Can you work these out from the model? Positions are in its coordinate system, mm. Coordinates: 2 decimals unless noted, no trailing zeros. Return JSON: item names as keys, results as strings. Group by question number.
1) For pin 1 Ø10 at (x, y) = (33.5, 26) entering from -Z; pin 2 Ø8 at (y, z) = (6, 452.5) entering from +X; pin 3 Ø13 at (x, z) = (-11, 514) entering from -Y, each with a flat end and sliding along its axis, tell me the tip position at first contact or that it passes through.
2) If I drill on line 1 along X through (y, z) = (-39, 925); line 2 along Y through (x, z) = (-5, 936.5); line 3 along Y through (x, z) = (28, 216.5), over which ranges is the centre line in solid material (lowest first)?
3) Imagine slicing it at A-A (z = 875). Give the number of separate pieces and of enclosed holes in the cut face, and give its area (3 significant figures).
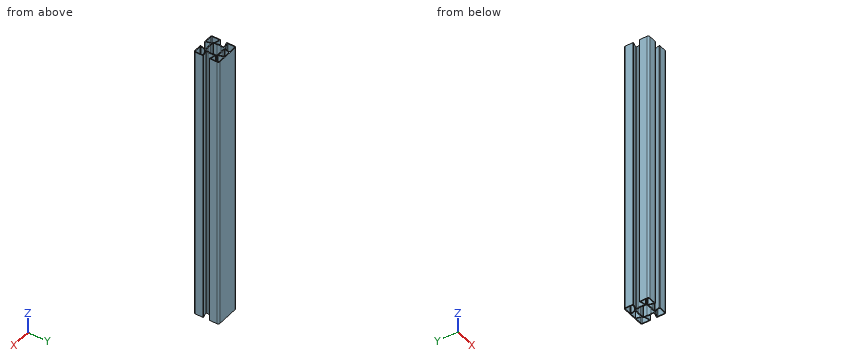
```python
from build123d import *

# Parameters (mm, degrees)
F1_DEPTH = 1000


# Not quite as in the source:
# - ends of sketch curves that miss each other by under 0.0002 mm in the source are joined


with BuildPart() as f1:
    # F0 (on Top) → F1 (new body)
    with BuildSketch(Plane.XY):
        with BuildLine():
            ThreePointArc((8.8614578186, -23.0888885991), (9.062799833, -23.022474706), (9.273618, -23))
            Line((9.273618, -23), (14.841657, -23))
            ThreePointArc((14.841657, -23), (15.6350103133, -23.3912385359), (15.8075828492, -24.2588189596))
            Line((15.8075828492, -24.2588189596), (10.671624, -43.426476))
            ThreePointArc((10.671624, -43.426476), (10.8873403242, -44.5109517857), (11.879032, -45))
            Line((11.879032, -45), (39, -45))
            ThreePointArc((39, -45), (43.2426406871, -43.2426406871), (45, -39))
            Line((45, -39), (45, -11.879032))
            ThreePointArc((45, -11.879032), (44.5109517857, -10.8873403242), (43.4264761923, -10.6716247175))
            Line((43.4264761923, -10.6716247175), (24.258819, -15.807583))
            ThreePointArc((24.258819, -15.807583), (23.3912385359, -15.6350103133), (23, -14.841657))
            Line((23, -14.841657), (23, -9.273618))
            ThreePointArc((23, -9.273618), (23.022474706, -9.062799833), (23.0888885991, -8.8614578186))
            ThreePointArc((23.0888885991, -8.8614578186), (25, 0), (23.0888887851, 8.8614579028))
            ThreePointArc((23.0888887851, 8.8614579028), (23.022474706, 9.062799833), (23, 9.273618))
            Line((23, 9.273618), (23, 14.841657))
            ThreePointArc((23, 14.841657), (23.3912385359, 15.6350103133), (24.2588189596, 15.8075828492))
            Line((24.2588189596, 15.8075828492), (43.426476, 10.671624))
            ThreePointArc((43.426476, 10.671624), (44.5109517857, 10.8873403242), (45, 11.879032))
            Line((45, 11.879032), (45, 39))
            ThreePointArc((45, 39), (43.2426406871, 43.2426406871), (39, 45))
            Line((39, 45), (-39, 45))
            ThreePointArc((-39, 45), (-43.2426406871, 43.2426406871), (-45, 39))
            Line((-45, 39), (-45, 11.879032))
            ThreePointArc((-45, 11.879032), (-44.5109517857, 10.8873403242), (-43.4264761923, 10.6716247175))
            Line((-43.4264761923, 10.6716247175), (-24.258819, 15.807583))
            ThreePointArc((-24.258819, 15.807583), (-23.3912385359, 15.6350103133), (-23, 14.841657))
            Line((-23, 14.841657), (-23, 9.273618))
            ThreePointArc((-23, 9.273618), (-23.022474706, 9.062799833), (-23.0888885991, 8.8614578186))
            ThreePointArc((-23.0888885991, 8.8614578186), (-25, 0), (-23.0888887851, -8.8614579028))
            ThreePointArc((-23.0888887851, -8.8614579028), (-23.022474706, -9.062799833), (-23, -9.273618))
            Line((-23, -9.273618), (-23, -14.841657))
            ThreePointArc((-23, -14.841657), (-23.3912385359, -15.6350103133), (-24.2588189596, -15.8075828492))
            Line((-24.2588189596, -15.8075828492), (-43.426476, -10.671624))
            ThreePointArc((-43.426476, -10.671624), (-44.5109517857, -10.8873403242), (-45, -11.879032))
            Line((-45, -11.879032), (-45, -39))
            ThreePointArc((-45, -39), (-43.2426406871, -43.2426406871), (-39, -45))
            Line((-39, -45), (-11.879032, -45))
            ThreePointArc((-11.879032, -45), (-10.8873403242, -44.5109517857), (-10.6716247175, -43.4264761923))
            Line((-10.6716247175, -43.4264761923), (-15.807583, -24.258819))
            ThreePointArc((-15.807583, -24.258819), (-15.6350103133, -23.3912385359), (-14.841657, -23))
            Line((-14.841657, -23), (-9.273618, -23))
            ThreePointArc((-9.273618, -23), (-9.062799833, -23.022474706), (-8.8614578186, -23.0888885991))
            ThreePointArc((-8.8614578186, -23.0888885991), (0, -25), (8.8614578186, -23.0888885991))
        make_face()
        with BuildLine():
            Line((-39.732362, -14.508469), (-24.482362, -18.594694))
            ThreePointArc((-24.482362, -18.594694), (-23.4132933733, -19.3090230718), (-23, -20.526546))
            Line((-23, -20.526546), (-23, -21))
            ThreePointArc((-23, -21), (-22.4142135624, -22.4142135624), (-21, -23))
            Line((-21, -23), (-20.526546, -23))
            ThreePointArc((-20.526546, -23), (-19.3090230718, -23.4132933733), (-18.5946943016, -24.4823620808))
            Line((-18.5946943016, -24.4823620808), (-14.508469, -39.732362))
            ThreePointArc((-14.508469, -39.732362), (-14.8536143733, -41.4675229282), (-16.440321, -42.25))
            Line((-16.440321, -42.25), (-39, -42.25))
            ThreePointArc((-39, -42.25), (-41.2980970389, -41.2980970389), (-42.25, -39))
            Line((-42.25, -39), (-42.25, -16.440321))
            ThreePointArc((-42.25, -16.440321), (-41.4675229282, -14.8536143733), (-39.732362, -14.508469))
        make_face(mode=Mode.SUBTRACT)
        with BuildLine():
            Line((14.508469, -39.732362), (18.594694, -24.482362))
            ThreePointArc((18.594694, -24.482362), (19.3090230718, -23.4132933733), (20.526546, -23))
            Line((20.526546, -23), (21, -23))
            ThreePointArc((21, -23), (22.4142135624, -22.4142135624), (23, -21))
            Line((23, -21), (23, -20.526546))
            ThreePointArc((23, -20.526546), (23.4132933733, -19.3090230718), (24.4823620808, -18.5946943016))
            Line((24.4823620808, -18.5946943016), (39.732362, -14.508469))
            ThreePointArc((39.732362, -14.508469), (41.4675229282, -14.8536143733), (42.25, -16.440321))
            Line((42.25, -16.440321), (42.25, -39))
            ThreePointArc((42.25, -39), (41.2980970389, -41.2980970389), (39, -42.25))
            Line((39, -42.25), (16.440321, -42.25))
            ThreePointArc((16.440321, -42.25), (14.8536143733, -41.4675229282), (14.508469, -39.732362))
        make_face(mode=Mode.SUBTRACT)
        with BuildLine():
            Line((-7.3951, -20.25), (-19.25, -20.25))
            ThreePointArc((-19.25, -20.25), (-19.9571067812, -19.9571067812), (-20.25, -19.25))
            Line((-20.25, -19.25), (-20.25, -7.3951))
            ThreePointArc((-20.25, -7.3951), (-20.2639867072, -7.2284333074), (-20.3055555728, -7.0664288513))
            ThreePointArc((-20.3055554887, -7.066428822), (-21.5, 0), (-20.3055554887, 7.066428822))
            ThreePointArc((-20.3055555728, 7.0664288513), (-20.2639867072, 7.2284333074), (-20.25, 7.3951))
            Line((-20.25, 7.3951), (-20.25, 19.25))
            ThreePointArc((-20.25, 19.25), (-19.9571067812, 19.9571067812), (-19.25, 20.25))
            Line((-19.25, 20.25), (-7.3951, 20.25))
            ThreePointArc((-7.3951, 20.25), (-7.2284333074, 20.2639867072), (-7.0664288513, 20.3055555728))
            ThreePointArc((-7.066428822, 20.3055554887), (0, 21.5), (7.066428822, 20.3055554887))
            ThreePointArc((7.0664288513, 20.3055555728), (7.2284333074, 20.2639867072), (7.3951, 20.25))
            Line((7.3951, 20.25), (19.25, 20.25))
            ThreePointArc((19.25, 20.25), (19.9571067812, 19.9571067812), (20.25, 19.25))
            Line((20.25, 19.25), (20.25, 7.3951))
            ThreePointArc((20.25, 7.3951), (20.2639867072, 7.2284333074), (20.3055555728, 7.0664288513))
            ThreePointArc((20.3055554887, 7.066428822), (21.5, 0), (20.3055554887, -7.066428822))
            ThreePointArc((20.3055555728, -7.0664288513), (20.2639867072, -7.2284333074), (20.25, -7.3951))
            Line((20.25, -7.3951), (20.25, -19.25))
            ThreePointArc((20.25, -19.25), (19.9571067812, -19.9571067812), (19.25, -20.25))
            Line((19.25, -20.25), (7.3951, -20.25))
            ThreePointArc((7.3951, -20.25), (7.2284333074, -20.2639867072), (7.0664288513, -20.3055555728))
            ThreePointArc((7.066428822, -20.3055554887), (0, -21.5), (-7.066428822, -20.3055554887))
            ThreePointArc((-7.0664288513, -20.3055555728), (-7.2284333074, -20.2639867072), (-7.3951, -20.25))
        make_face(mode=Mode.SUBTRACT)
        with BuildLine():
            Line((-14.508469, 39.732362), (-18.594694, 24.482362))
            ThreePointArc((-18.594694, 24.482362), (-19.3090230718, 23.4132933733), (-20.526546, 23))
            Line((-20.526546, 23), (-21, 23))
            ThreePointArc((-21, 23), (-22.4142135624, 22.4142135624), (-23, 21))
            Line((-23, 21), (-23, 20.526546))
            ThreePointArc((-23, 20.526546), (-23.4132933733, 19.3090230718), (-24.4823620808, 18.5946943016))
            Line((-24.4823620808, 18.5946943016), (-39.732362, 14.508469))
            ThreePointArc((-39.732362, 14.508469), (-41.4675229282, 14.8536143733), (-42.25, 16.440321))
            Line((-42.25, 16.440321), (-42.25, 39))
            ThreePointArc((-42.25, 39), (-41.2980970389, 41.2980970389), (-39, 42.25))
            Line((-39, 42.25), (-16.440321, 42.25))
            ThreePointArc((-16.440321, 42.25), (-14.8536143733, 41.4675229282), (-14.508469, 39.732362))
        make_face(mode=Mode.SUBTRACT)
        with BuildLine():
            Line((-9.273618, 23), (-14.841657, 23))
            ThreePointArc((-14.841657, 23), (-15.6350103133, 23.3912385359), (-15.8075828492, 24.2588189596))
            Line((-15.8075828492, 24.2588189596), (-10.98686, 42.25))
            Line((-10.98686, 42.25), (10.98686, 42.25))
            Line((10.98686, 42.25), (15.807583, 24.258819))
            ThreePointArc((15.807583, 24.258819), (15.6350103133, 23.3912385359), (14.841657, 23))
            Line((14.841657, 23), (9.273618, 23))
            ThreePointArc((9.273618, 23), (9.062799833, 23.022474706), (8.8614578186, 23.0888885991))
            ThreePointArc((8.8614578186, 23.0888885991), (0, 25), (-8.8614579028, 23.0888887851))
            ThreePointArc((-8.8614579028, 23.0888887851), (-9.062799833, 23.022474706), (-9.273618, 23))
        make_face(mode=Mode.SUBTRACT)
        with BuildLine():
            Line((39.732362, 14.508469), (24.482362, 18.594694))
            ThreePointArc((24.482362, 18.594694), (23.4132933733, 19.3090230718), (23, 20.526546))
            Line((23, 20.526546), (23, 21))
            ThreePointArc((23, 21), (22.4142135624, 22.4142135624), (21, 23))
            Line((21, 23), (20.526546, 23))
            ThreePointArc((20.526546, 23), (19.3090230718, 23.4132933733), (18.5946943016, 24.4823620808))
            Line((18.5946943016, 24.4823620808), (14.508469, 39.732362))
            ThreePointArc((14.508469, 39.732362), (14.8536143733, 41.4675229282), (16.440321, 42.25))
            Line((16.440321, 42.25), (39, 42.25))
            ThreePointArc((39, 42.25), (41.2980970389, 41.2980970389), (42.25, 39))
            Line((42.25, 39), (42.25, 16.440321))
            ThreePointArc((42.25, 16.440321), (41.4675229282, 14.8536143733), (39.732362, 14.508469))
        make_face(mode=Mode.SUBTRACT)
    extrude(amount=F1_DEPTH)


solid = f1.part
```
Calculated:
{
 "1": {"pin 1": "through", "pin 2": "x = 24.91", "pin 3": "y = -45"},
 "2": {"line 1": "-45 to -42.25, -14.7 to -11.86, 11.86 to 14.7, 42.25 to 45", "line 2": "-24.41 to -20.91, 20.91 to 24.41, 42.25 to 45", "line 3": "-45 to -42.25, -17.65 to -14.81, 14.81 to 17.65, 42.25 to 45"},
 "3": {"separate pieces": "1", "enclosed holes": "6", "area": "1,740 mm2"}
}
